The model under review builds one solid part; all positions refer to its coordinate system, in mm. Face numbers are marked on the shaded views. Coordinates: 2 decimals unless noted, no trailing zeros. Loops run counter-clockwise (first coordinate to the right, second up) from the corner with the lowest first, then second, coordinate; pieces in that order, holes last. Notation, with made-up numbers: (-29.75, 24.5) - (24.25, 24.5) arc R15 ccw to (24.25, 40.5) - close; hole circle Ø8 at (40.25, -31). An arc over 180 degrees is marked (long way). One line per item, written item: value. Start each with the question number.
1. To check wall thickness, follow line 1 (Z direction, x = -3.5, y = 21); line 2 (Y direction, x = -6.5, z = 18.5); line 3 (Z direction, x = -11, y = -17). State the ranges of each line that lie inside material, in increasing order.
2. Insertion check: P1, Ø10, axis at y = -10, z = 9.5, coming from the -X side; P2, Ø3.5, axis at y = -16.97, z = -16.97, coming from the -X side; P3, Ø4, axis at x = -7, y = 2, coming from the -Z side; P4, Ø5, axis at x = -26.5, y = -3, coming from the -Z side. Each pin has a flat end and moves straight along its axis. Give the tip position at first contact, or say it passes through.
3. We need section D-D, the plane z = 25. Give the boundary of the cut face in (x, y).
4. We need section A-A, the plane y = 13.5. Give the boundary of the cut face in (x, z), then the cut area to 3 significant figures.
5. We need section C-C, the plane x = -4. Give the boundary of the cut face in (y, z).
6. We need section B-B, the plane x = -16. Give the boundary of the cut face in (y, z).
7. Mouldability with a two-part tool opening along Y and no side actions: class the marked faces 1, 2 and 3 as +Y half, -Y half, draft (parallel to the pull), parting line (faces both ways), or undercut.
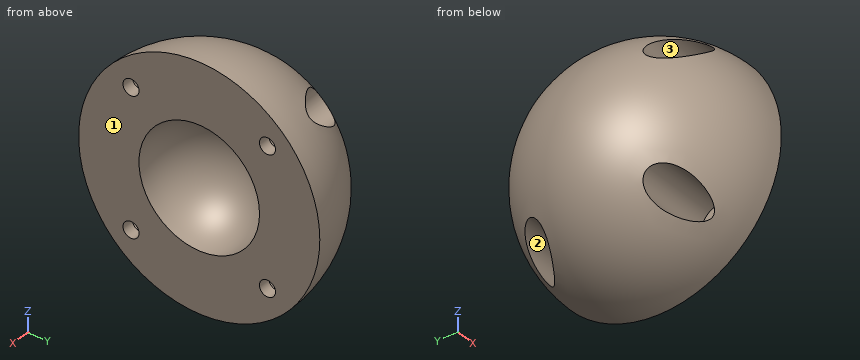
from build123d import *

# Parameters (mm, degrees)
SKETCH4_R               = 2
CUT_EXTRUDE3_DEPTH      = 1
CUT_EXTRUDE3_DEPTH_BACK = 31
SKETCH5_R               = 4.5
CUT_EXTRUDE4_DEPTH      = 28


with BuildPart() as part:
    # Sketch3 → Revolve1 (revolve)
    with BuildSketch(Plane.XY):
        with BuildLine():
            Line((-30, 0), (-15, 0))
            ThreePointArc((-15, 0), (-10.606601718, 10.606601718), (0, 15))
            Line((0, 15), (0, 30))
            ThreePointArc((0, 30), (-21.213203436, 21.213203436), (-30, 0))
        make_face()
    revolve(axis=Axis((0, 0, 0), (-1, 0, 0)))

    # Sketch4 → Cut-Extrude3 (cut, two sides)
    with BuildSketch(Plane(origin=(0, 0, 0), x_dir=(0, 0, -1), z_dir=(1, 0, 0))) as cut_extrude3_sk:
        with Locations((-16.970562748, 16.970562748)):
            Circle(SKETCH4_R)
        with Locations((16.970562748, 16.970562748)):
            Circle(SKETCH4_R)
        with Locations((16.970562748, -16.970562748)):
            Circle(SKETCH4_R)
        with Locations((-16.970562748, -16.970562748)):
            Circle(SKETCH4_R)
    extrude(amount=CUT_EXTRUDE3_DEPTH, mode=Mode.SUBTRACT)
    extrude(cut_extrude3_sk.sketch, amount=-CUT_EXTRUDE3_DEPTH_BACK, mode=Mode.SUBTRACT)

    # Sketch5 → Cut-Extrude4 (cut, through all)
    with BuildSketch(Plane(origin=(-3, 0, 0), x_dir=(0, 0, -1), z_dir=(1, 0, 0))):
        with Locations((-16.970562748, 16.970562748)):
            Circle(SKETCH5_R)
        with Locations((16.970562748, 16.970562748)):
            Circle(SKETCH5_R)
        with Locations((16.970562748, -16.970562748)):
            Circle(SKETCH5_R)
        with Locations((-16.970562748, -16.970562748)):
            Circle(SKETCH5_R)
    extrude(amount=-CUT_EXTRUDE4_DEPTH, mode=Mode.SUBTRACT)


solid = part.part
Findings below:
1. line 1: -21.14 to -18.97, -14.97 to 14.97, 18.97 to 21.14
1. line 2: -22.7 to -21.2, -12.74 to 12.74, 21.2 to 22.7
1. line 3: -22.14 to -21.47, -12.47 to 12.47, 21.47 to 22.14
2. P1: x = -28.68
2. P2: through
2. P3: z = -29.53
2. P4: z = -17.77
3. outline: (0, -16.58) - (0, 16.58) arc R16.58 ccw to start
4. outline: (-22.78, -14.11) - (-3, -14.11) - (-3, -19.84) - (-18.01, -19.84) arc R26.79 ccw to (0, -26.79) - (0, -6.54) arc R6.54 cw to (0, 6.54) - (0, 26.79) arc R26.79 ccw to (-18.01, 19.84) - (-3, 19.84) - (-3, 14.11) - (-22.78, 14.11) arc R26.79 ccw to start
4. area: 858 mm2
5. outline: circle Ø59.46 at (0, 0); hole circle Ø9 at (-16.97, -16.97); hole circle Ø9 at (-16.97, 16.97); hole circle Ø28.91 at (0, 0); hole circle Ø9 at (16.97, -16.97); hole circle Ø9 at (16.97, 16.97)
6. outline: (-20.78, -14.57) arc R4.5 cw (long way) to (-14.57, -20.78) arc R25.38 ccw to (14.57, -20.78) arc R4.5 cw (long way) to (20.78, -14.57) arc R25.38 ccw to (20.78, 14.57) arc R4.5 cw (long way) to (14.57, 20.78) arc R25.38 ccw to (-14.57, 20.78) arc R4.5 cw (long way) to (-20.78, 14.57) arc R25.38 ccw to start
7. face 1: draft
7. face 2: undercut
7. face 3: undercut
